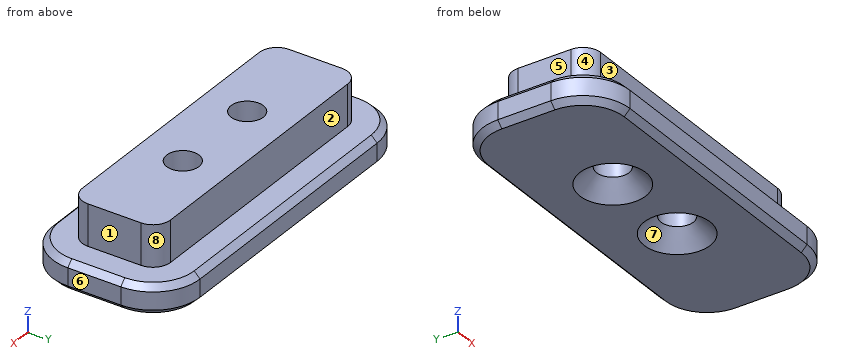
```python
from build123d import *

# Parameters (mm, degrees)
F0_W           = 50
F0_H           = 15
F1_DEPTH       = 7
F2_W           = 60
F2_H           = 25
F2_W_2         = 50
F2_H_2         = 15
F3_DEPTH       = 5
F5_D           = 5.5
F5_CSINK_D     = 11.2
F5_CSINK_ANGLE = 90
F6_R           = 8
F7_R           = 3
F8_SIZE        = 1


with BuildPart() as f1:
    # F0 (on Top) → F1 (new body)
    with BuildSketch(Plane.XY):
        Rectangle(F0_W, F0_H)
    extrude(amount=F1_DEPTH)

    # F2 (on face) → F3 (join)
    with BuildSketch(Plane(origin=(0, 0, 0), x_dir=(1, 0, 0), z_dir=(0, 0, -1))):
        Rectangle(F2_W, F2_H)
        Rectangle(F2_W_2, F2_H_2, mode=Mode.SUBTRACT)
        Rectangle(F2_W_2, F2_H_2)
    extrude(amount=F3_DEPTH)

    # F5 (through all)
    with Locations(Plane(origin=(0, 0, -5), x_dir=(1, 0, 0), z_dir=(0, 0, -1))):
        with Locations((-8, 0), (8, 0)):
            CounterSinkHole(F5_D / 2, F5_CSINK_D / 2, counter_sink_angle=F5_CSINK_ANGLE)

    # F6
    f6_edges = [f1.edges().sort_by_distance(p)[0] for p in [
        (-30, -12.5, -2.5),
        (-30, 12.5, -2.5),
        (30, -12.5, -2.5),
        (30, 12.5, -2.5),
    ]]
    fillet(f6_edges, radius=F6_R)

    # F7
    f7_edges = [f1.edges().sort_by_distance(p)[0] for p in [
        (25, -7.5, 3.5),
        (25, 7.5, 3.5),
        (-25, 7.5, 3.5),
        (-25, -7.5, 3.5),
    ]]
    fillet(f7_edges, radius=F7_R)

    # F8
    f8_edges = [f1.edges().sort_by_distance(p)[0] for p in [
        (0, -12.5, -5),
        (30, 0, -5),
        (0, 12.5, -5),
        (-30, 0, -5),
        (-30, 0, 0),
        (0, 12.5, 0),
        (30, 0, 0),
        (0, -12.5, 0),
    ]]
    chamfer(f8_edges, length=F8_SIZE)


solid = f1.part
```
Input: part model. Units: mm. Frame: model coordinates. Face numbers are marked on the shaded views. A direction names the side the tool comes from. Round coordinates to 2 decimals unless told otherwise and drop trailing zeros. Write each loop counter-clockwise with the first axis right and the second up, starting at its lowest first coordinate (ties: lowest second). Pieces come first, ordered by that corner, then holes. Notation, with made-up numbers: (37.5, 59.5) - (94.5, 59.5) arc R32 ccw to (94.5, 95.5) - close; hole circle Ø5 at (-7, 25.5). An arc over 180 degrees is marked (long way). Write item = value, one per line.
(1) Material intervals for probe 1 along Y at (x, z) = (-8, 2); probe 2 along X at (y, z) = (-0.25, 5.5); probe 3 along X at (y, z) = (2.5, -2), sorted ascending.
Geometry check:
probe_1 = -7.5 to -2.75, 2.75 to 7.5
probe_2 = -25 to -10.74, -5.26 to 5.26, 10.74 to 25
probe_3 = -30 to -9.15, -6.85 to 6.85, 9.15 to 30
(2) Section query B-B on x = 8. Output: boundary loops of the cut face in (y, z).
Geometry check:
outline = (-12.5, -4) - (-11.5, -5) - (-5.6, -5) - (-2.75, -2.15) - (-2.75, 7) - (-7.5, 7) - (-7.5, 0) - (-11.5, 0) - (-12.5, -1) - close; (2.75, -2.15) - (5.6, -5) - (11.5, -5) - (12.5, -4) - (12.5, -1) - (11.5, 0) - (7.5, 0) - (7.5, 7) - (2.75, 7) - close
(3) Section query D-D on x = -19.5. Output: boundary loops of the cut face in (y, z).
Geometry check:
outline = (-12.5, -4) - (-11.5, -5) - (11.5, -5) - (12.5, -4) - (12.5, -1) - (11.5, 0) - (7.5, 0) - (7.5, 7) - (-7.5, 7) - (-7.5, 0) - (-11.5, 0) - (-12.5, -1) - close
(4) Contact query for flat-ended pins moving along their axis: pin 1 Ø5.5 at (x, z) = (3, 5) entering from +Y; pin 2 Ø3.5 at (y, z) = (1.5, 2.5) entering from +X; pin 3 Ø4 at (y, z) = (-9, 1.5) entering from -X; pin 4 Ø12 at (x, y) = (22, -9.5) entering from +Z. Output: stop coordinate, or through.
Geometry check:
pin_1 = 7.5
pin_2 = 25
pin_3 = -28.33
pin_4 = 7
(5) Pull-direction query (Y, two-part tool) for the marked faces 6, 7 and 8; classes: +Y half, -Y half, draft (parallel to the pull), parting line (faces both ways), or undercut.
Geometry check:
face_6 = draft
face_7 = undercut
face_8 = +Y half
(6) Section query C-C on y = 0. Output: boundary loops of the cut face in (x, z), then the cut area to 3 significant figures.
Geometry check:
outline = (-30, -4) - (-29, -5) - (-13.6, -5) - (-10.75, -2.15) - (-10.75, 7) - (-25, 7) - (-25, 0) - (-29, 0) - (-30, -1) - close; (-5.25, -2.15) - (-2.4, -5) - (2.4, -5) - (5.25, -2.15) - (5.25, 7) - (-5.25, 7) - close; (10.75, -2.15) - (13.6, -5) - (29, -5) - (30, -4) - (30, -1) - (29, 0) - (25, 0) - (25, 7) - (10.75, 7) - close
area = 500 mm^2
(7) Access query for the marked faces 1, 2, 3, 4 and 5. Directions: +Z, -Z, +X, -X, +Y, -Y. A direction counts if a zero-diameter tool reaches every point of the face in a straight line with its end or side. Return the directions, or none.
Geometry check:
face_1 = +Z, +X, +Y, -Y
face_2 = +Z, +X, -X, +Y
face_3 = +Z, +X, -X, -Y
face_4 = +Z, -X, -Y
face_5 = +Z, -X, +Y, -Y
(8) Section query A-A on z = 4.25. Output: boundary loops of the cut face in (x, y).
Geometry check:
outline = (-25, -4.5) arc R3 ccw to (-22, -7.5) - (22, -7.5) arc R3 ccw to (25, -4.5) - (25, 4.5) arc R3 ccw to (22, 7.5) - (-22, 7.5) arc R3 ccw to (-25, 4.5) - close; hole circle Ø5.5 at (-8, 0); hole circle Ø5.5 at (8, 0)
